```python
from build123d import *

# Parameters (mm, degrees)
PAD_DEPTH = 6


with BuildPart() as part:
    # Sketch → Pad (new body)
    with BuildSketch(Plane.XY):
        with BuildLine():
            ThreePointArc((-20, 22.36068), (0, -30), (20, 22.36068))
            Line((20, 22.36068), (19.400305, 36.34783))
            Line((19.400305, 36.34783), (8.749783, 25.182296))
            ThreePointArc((8.749783, 25.182296), (0, 26.659084), (-8.749783, 25.182296))
            Line((-19.400305, 36.34783), (-8.749783, 25.182296))
            Line((-20, 22.36068), (-19.400305, 36.34783))
        make_face()
    extrude(amount=-PAD_DEPTH)


solid = part.part
```
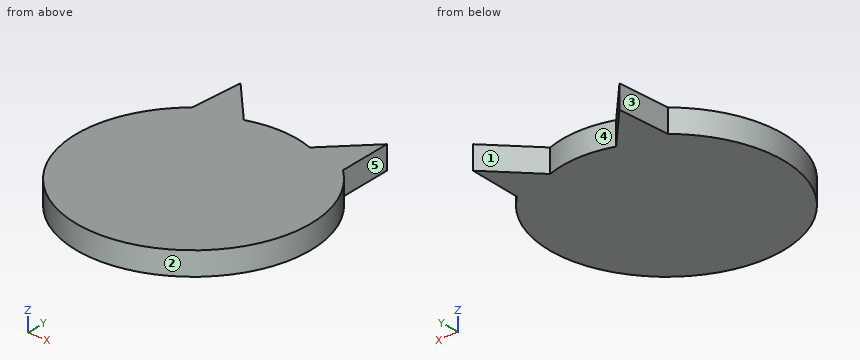
Read the model definition and answer for the solid it produces. Units are mm, in the model's axes. Face numbers are marked on the shaded views. A direction names the side the tool comes from. Coordinates: 2 decimals unless noted, no trailing zeros. Order: outer loops, then holes, each group sorted by start corner. A loop starts at its lowest first (then second) coordinate and runs counter-clockwise, first axis right, second up. Notation, with made-up numbers: (14, 24.5) - (68, 24.5) arc R24 ccw to (68, 42.5) - close; hole circle Ø11 at (15.5, 15.5). An arc over 180 degrees is marked (long way). Answer as a JSON object with one key per item and string values. Group by question number.
Item 1: The mould has two halves that part along X. Classify the marked faces 3, 4 and 5: +X half, -X half, draft (parallel to the pull), parting line (faces both ways), or undercut.
Item 2: Section C-C (y = 13) is taken. Give the vertices of the cut face in (x, z).
Item 3: Flat-ended cylindrical pins translate along their axes: P1, Ø3, axis at x = -1, z = -1, coming from the +Y side; P2, Ø2, axis at x = 9, z = -4, coming from the -Y side; P3, Ø1, axis at y = 22, z = -2.5, coming from the -X side. Find the tip coordinate at first contact, or state that the pin passes through.
Item 4: Consider probe 1 along X at (y, z) = (33, -0.7); probe 2 along X at (y, z) = (-1, -2.55); probe 3 along Y at (x, z) = (26.5, -3.1). Determine where each line is inside the solid, lowest interval first. Write a range as from..to.
Item 5: Section A-A (z = -3.6) is taken. Give the vertices of the cut face in (x, y), plus the area to 3 significant figures.
Item 6: Section B-B (x = 0) is taken. Give the vertices of the cut face in (y, z), plus the area to 3 significant figures.
Item 7: A tool of negligible diameter and unlimited length cuts with its end or side. For the marked faces 1 and 2, from which of +Z, -Z, +X, -X, +Y, -Y can it reach the whole face along a straight path? Write none if from no direction.
Results are:
{
 "1": {"face 3": "-X half", "face 4": "undercut", "face 5": "+X half"},
 "2": {"outline": "(-27.04, -6) - (27.04, -6) - (27.04, 0) - (-27.04, 0) - close"},
 "3": {"P1": "stops at y = 26.66", "P2": "stops at y = -28.91", "P3": "stops at x = -20.92"},
 "4": {"probe 1": "x = -19.54..-16.21, 16.21..19.54", "probe 2": "x = -29.98..29.98", "probe 3": "y = -14.06..14.06"},
 "5": {"outline": "(-20, 22.36) arc R30 ccw (long way) to (20, 22.36) - (19.4, 36.35) - (8.75, 25.18) arc R26.66 ccw to (-8.75, 25.18) - (-19.4, 36.35) - close", "area": "2,870 mm^2"},
 "6": {"outline": "(-30, -6) - (26.66, -6) - (26.66, 0) - (-30, 0) - close", "area": "340 mm^2"},
 "7": {"face 1": "+Z, -Z, +Y", "face 2": "+Z, -Z"}
}
